Could you check a few things on this model? Use its own coordinates, in mm. Face numbers are marked on the shaded views. Give positions to 0.01 mm unless a question says otherwise; leave off trailing zeros. Order: outer loops, then holes, each group sorted by start corner. A loop starts at its lowest first (then second) coordinate and runs counter-clockwise, first axis right, second up.
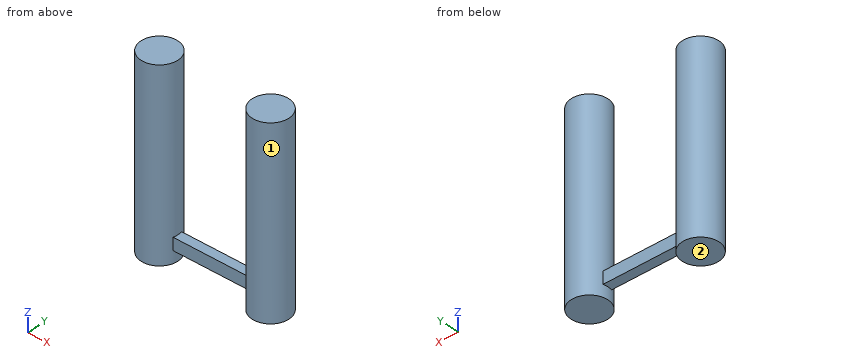
from build123d import *

# Parameters (mm, degrees)
F1_W     = 13.079472
F1_H     = 16.876735
F2_DEPTH = 76.2
F0_R     = 25.4
F3_DEPTH = 254


with BuildPart() as f2:
    # F1 (on Right) → F2 (new body, symmetric)
    with BuildSketch(Plane.YZ):
        with Locations((6e-06, 24.893183)):
            Rectangle(F1_W, F1_H)
    extrude(amount=F2_DEPTH, both=True)

    # F0 (on Top) → F3 (join)
    with BuildSketch(Plane.XY):
        with Locations((-76.2, 0)):
            Circle(F0_R)
        with Locations((76.2, 0)):
            Circle(F0_R)
    extrude(amount=F3_DEPTH)


solid = f2.part
Item 1: Imagine slicing it at B-B on z = 150. List the corners of the cut face in (x, y) for me.
Findings:
outline: circle Ø50.8 at (-76.2, 0); circle Ø50.8 at (76.2, 0)
Item 2: Imagine slicing it at D-D on y = -15. List the corners of the cut face in (x, z) for me, then the cut area to 3 significant figures.
Findings:
outline: (-96.7, 0) - (-55.7, 0) - (-55.7, 254) - (-96.7, 254) - close; (55.7, 0) - (96.7, 0) - (96.7, 254) - (55.7, 254) - close
area: 20,800 mm2
Item 3: Imagine slicing it at A-A on y = 17.5. List the corners of the cut face in (x, z) for me.
Findings:
outline: (-94.61, 0) - (-57.79, 0) - (-57.79, 254) - (-94.61, 254) - close; (57.79, 0) - (94.61, 0) - (94.61, 254) - (57.79, 254) - close
Item 4: We'd pull the mould along X, two halves only. Please class the marked faces 1 and 2: +X half, -X half, draft (parallel to the pull), parting line (faces both ways), or undercut.
Findings:
face 1: undercut
face 2: draft
Item 5: For pin 1 (6 mm diameter, centred on x = -76, z = 74, fed in from -Y); pin 2 (6 mm diameter, centred on y = 13, z = 107, fed in from +X); pin 3 (2 mm diameter, centred on y = 20, z = 171.5, fed in from -X), each with a flat end and sliding along its axis, tell me the tip position at first contact or that it passes through.
Findings:
pin 1: stops at y = -25.4
pin 2: stops at x = 99.55
pin 3: stops at x = -93.06
Item 6: Please list where these lines run through material, in increasing order: line 1 along Z through (x, y) = (-44.5, 5); line 2 along X through (y, z) = (-10.5, 121.5); line 3 along X through (y, z) = (11, 201.5).
Findings:
line 1: z = 16.45 to 33.33
line 2: x = -99.33 to -53.07, 53.07 to 99.33
line 3: x = -99.09 to -53.31, 53.31 to 99.09
Item 7: Imagine slicing it at C-C on y = 0. List the corners of the cut face in (x, z) for me, then the cut area to 3 significant figures.
Findings:
outline: (-101.6, 0) - (-50.8, 0) - (-50.8, 16.45) - (50.8, 16.45) - (50.8, 0) - (101.6, 0) - (101.6, 254) - (50.8, 254) - (50.8, 33.33) - (-50.8, 33.33) - (-50.8, 254) - (-101.6, 254) - close
area: 27,500 mm2
